```python
from build123d import *

# Parameters (mm, degrees)
F1_DEPTH = 206.502
F2_W     = 189.611
F2_H     = 103.378
F3_DEPTH = 25.4
F4_W     = 189.611
F4_H     = 101.6
F5_DEPTH = 25.4


with BuildPart() as f1:
    # F0 (on Right) → F1 (new body)
    with BuildSketch(Plane.YZ):
        with BuildLine():
            Line((432.308, 0), (1.778, 0))
            ThreePointArc((1.778, 0), (0.520764, -0.520764), (0, -1.778))
            Line((0, -1.778), (0, -129.286))
            Line((0, -129.286), (2.032, -129.286))
            Line((2.032, -129.286), (2.032, -2.032))
            Line((2.032, -2.032), (432.054, -2.032))
            Line((432.054, -2.032), (432.054, -129.286))
            Line((432.054, -129.286), (434.086, -129.286))
            Line((434.086, -129.286), (434.086, -1.778))
            ThreePointArc((434.086, -1.778), (433.565236, -0.520764), (432.308, 0))
        make_face()
    extrude(amount=F1_DEPTH)

    # F2 (on face) → F3 (cut)
    with BuildSketch(Plane.XZ):
        with Locations((100.6729, -65.659)):
            Rectangle(F2_W, F2_H)
    extrude(amount=-F3_DEPTH, mode=Mode.SUBTRACT)

    # F4 (on face) → F5 (cut)
    with BuildSketch(Plane(origin=(0, 434.086, 0), x_dir=(-1, 0, 0), z_dir=(0, 1, 0))):
        with Locations((-100.6729, -66.548)):
            Rectangle(F4_W, F4_H)
    extrude(amount=-F5_DEPTH, mode=Mode.SUBTRACT)


solid = f1.part
```
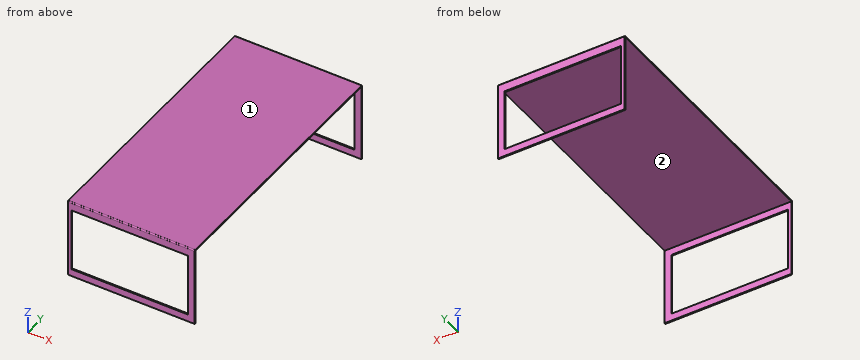
Check sheet for the modelled part. Datum: model origin and axes. Units: mm. Face numbers are marked on the shaded views. Round coordinates to 2 decimals unless told otherwise and drop trailing zeros. Order: outer loops, then holes, each group sorted by start corner. A loop starts at its lowest first (then second) coordinate and runs counter-clockwise, first axis right, second up. Notation, with made-up numbers: M 42.25,21 L 82.25,21 A27 cw 82.25,45 Z; hole C -20,20.25 d11. An arc over 180 degrees is marked long. Answer in a Markdown table with one row per item.
(1) Draft check along Y on the marked faces 1 and 2. Enter one of: +Y half, -Y half, draft (parallel to the pull), parting line (faces both ways), or undercut.
Findings:
| item | result |
|---|---|
| face 1 | draft |
| face 2 | undercut |
(2) Section check A-A on z = -52. Record the boundary of the cut face in (x, y).
Findings:
| item | result |
|---|---|
| outline | M 0,0 L 5.87,0 L 5.87,2.03 L 0,2.03 Z; M 0,432.05 L 5.87,432.05 L 5.87,434.09 L 0,434.09 Z; M 195.48,0 L 206.5,0 L 206.5,2.03 L 195.48,2.03 Z; M 195.48,432.05 L 206.5,432.05 L 206.5,434.09 L 195.48,434.09 Z |
(3) Section check C-C on y = 35. Record the boundary of the cut face in (x, z).
Findings:
| item | result |
|---|---|
| outline | M 0,-2.03 L 206.5,-2.03 L 206.5,0 L 0,0 Z |
(4) Material ranges on line 1 along Y through (x, z) = (183.5, -13.5); line 2 along Z through (x, y) = (39.5, 270.5), recorded low to high. Write a range as from..to.
Findings:
| item | result |
|---|---|
| line 1 | y = 0..2.03, 432.05..434.09 |
| line 2 | z = -2.03..0 |
(5) Gauge pin test, flat ends, axial feed: pin 1 (1 mm diameter, centred on x = 101.5, y = 433, fed in from +Z); pin 2 (1.6 mm diameter, centred on y = 433, z = -48.5, fed in from -X); pin 3 (8 mm diameter, centred on x = 154, y = 57.5, fed in from -Z); pin 4 (1.6 mm diameter, centred on x = 71.5, y = 0.5, fed in from +Z). Record the tip position at first contact, or that the pin passes through.
Findings:
| item | result |
|---|---|
| pin 1 | stops at z = -0.01 |
| pin 2 | stops at x = 0 |
| pin 3 | stops at z = -2.03 |
| pin 4 | stops at z = -0.07 |
(6) Section check B-B on x = 148. Record the boundary of the cut face in (y, z).
Findings:
| item | result |
|---|---|
| outline | M 0,-129.29 L 2.03,-129.29 L 2.03,-117.35 L 0,-117.35 Z; M 0,-13.97 L 2.03,-13.97 L 2.03,-2.03 L 432.05,-2.03 L 432.05,-15.75 L 434.09,-15.75 L 434.09,-1.78 A1.78 ccw 432.31,0 L 1.78,0 A1.78 ccw 0,-1.78 Z; M 432.05,-129.29 L 434.09,-129.29 L 434.09,-117.35 L 432.05,-117.35 Z |
